```python
from build123d import *

# Parameters (mm, degrees)
F1_DEPTH = 3


with BuildPart() as f1:
    # F0 (on Front) → F1 (new body)
    with BuildSketch(Plane.XZ):
        Polygon((152.04934, 116.75), (152.04934, 119.75), (136.84934, 119.75), (136.84934, 116.75), (121.64934, 116.75), (121.64934, 119.75), (106.44934, 119.75), (106.44934, 116.75), (91.24934, 116.75), (91.24934, 119.75), (76.04934, 119.75), (76.04934, 116.75), (60.84934, 116.75), (60.84934, 119.75), (45.64934, 119.75), (45.64934, 116.75), (30.44934, 116.75), (30.44934, 119.75), (15.24934, 119.75), (15.24934, 116.75), (0.04934, 116.75), (-0.04934, 116.75), (-0.04934, 119.75), (-15.24934, 119.75), (-15.24934, 116.75), (-30.44934, 116.75), (-30.44934, 119.75), (-45.64934, 119.75), (-45.64934, 116.75), (-60.84934, 116.75), (-60.84934, 119.75), (-76.04934, 119.75), (-76.04934, 116.75), (-91.24934, 116.75), (-91.24934, 119.75), (-106.44934, 119.75), (-106.44934, 116.75), (-121.64934, 116.75), (-121.64934, 119.75), (-136.84934, 119.75), (-136.84934, 116.75), (-152.04934, 116.75), (-152.04934, 119.75), (-167.24934, 119.75), (-167.24934, 106.45), (-164.24934, 106.45), (-164.24934, 93.15), (-167.24934, 93.15), (-167.24934, 79.85), (-164.24934, 79.85), (-164.24934, 66.55), (-167.24934, 66.55), (-167.24934, 53.25), (-164.24934, 53.25), (-164.24934, 39.95), (-167.24934, 39.95), (-167.24934, 26.65), (-164.24934, 26.65), (-164.24934, 13.35), (-167.24934, 13.35), (-167.24934, 0.05), (-164.24934, 0.05), (-164.24934, -0.05), (-164.24934, -13.35), (-167.24934, -13.35), (-167.24934, -26.65), (-164.24934, -26.65), (-164.24934, -39.95), (-167.24934, -39.95), (-167.24934, -53.25), (-164.24934, -53.25), (-164.24934, -66.55), (-167.24934, -66.55), (-167.24934, -79.85), (-164.24934, -79.85), (-164.24934, -93.15), (-167.24934, -93.15), (-167.24934, -106.45), (-164.24934, -106.45), (-164.24934, -119.75), (-152.04934, -119.75), (-152.04934, -116.75), (-136.84934, -116.75), (-136.84934, -119.75), (-121.64934, -119.75), (-121.64934, -116.75), (-106.44934, -116.75), (-106.44934, -119.75), (-91.24934, -119.75), (-91.24934, -116.75), (-76.04934, -116.75), (-76.04934, -119.75), (-60.84934, -119.75), (-60.84934, -116.75), (-45.64934, -116.75), (-45.64934, -119.75), (-30.44934, -119.75), (-30.44934, -116.75), (-15.24934, -116.75), (-15.24934, -119.75), (-0.04934, -119.75), (-0.04934, -116.75), (0.04934, -116.75), (15.24934, -116.75), (15.24934, -119.75), (30.44934, -119.75), (30.44934, -116.75), (45.64934, -116.75), (45.64934, -119.75), (60.84934, -119.75), (60.84934, -116.75), (76.04934, -116.75), (76.04934, -119.75), (91.24934, -119.75), (91.24934, -116.75), (106.44934, -116.75), (106.44934, -119.75), (121.64934, -119.75), (121.64934, -116.75), (136.84934, -116.75), (136.84934, -119.75), (152.04934, -119.75), (152.04934, -116.75), (164.24934, -116.75), (164.24934, -106.45), (167.24934, -106.45), (167.24934, -93.15), (164.24934, -93.15), (164.24934, -79.85), (167.24934, -79.85), (167.24934, -66.55), (164.24934, -66.55), (164.24934, -53.25), (167.24934, -53.25), (167.24934, -39.95), (164.24934, -39.95), (164.24934, -26.65), (167.24934, -26.65), (167.24934, -13.35), (164.24934, -13.35), (164.24934, -0.05), (164.24934, 0.05), (167.24934, 0.05), (167.24934, 13.35), (164.24934, 13.35), (164.24934, 26.65), (167.24934, 26.65), (167.24934, 39.95), (164.24934, 39.95), (164.24934, 53.25), (167.24934, 53.25), (167.24934, 66.55), (164.24934, 66.55), (164.24934, 79.85), (167.24934, 79.85), (167.24934, 93.15), (164.24934, 93.15), (164.24934, 106.45), (167.24934, 106.45), (167.24934, 116.75), align=None)
    extrude(amount=F1_DEPTH)


solid = f1.part
```
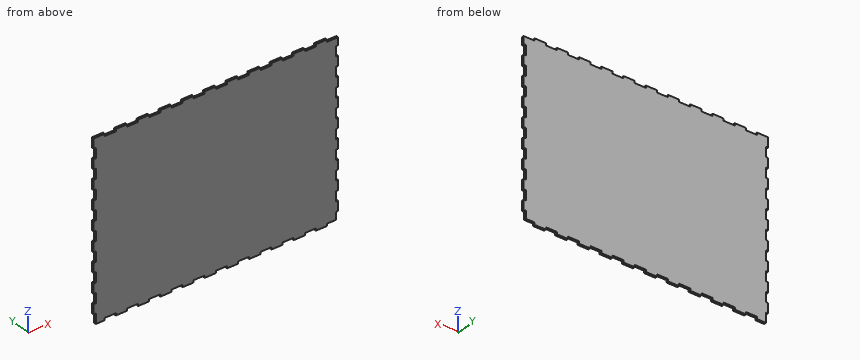
Geometry: final body of the model. Coordinates: model frame, mm. Coordinates: 2 decimals unless noted, no trailing zeros. Loops run counter-clockwise (first coordinate to the right, second up) from the corner with the lowest first, then second, coordinate; pieces in that order, holes last. Notation, with made-up numbers: (48.25, 44) -> (93.25, 44) arc R19 cw to (93.25, 72) -> close; hole circle Ø5 at (-30, 83.5). An arc over 180 degrees is marked (long way). Use a Markdown table: item, result. Add a question column.
(1) Section query A-A, the plane z = -59.5. Return loops of the section in (x, y), plus the area to 3 significant figures.
(2) Pin query (flat end, axial travel): pin 1 Ø1.5 at (x, y) = (-82.5, -1) entering from -Z; pin 2 Ø1.5 at (y, z) = (-2, -119) entering from -X; pin 3 Ø0.9 at (y, z) = (-1, 118) entering from +X. Return the tip coordinate at first contact, or that it passes through.
(3) Line query: line 1 along X through (y, z) = (-1.55, 104.5); line 2 along Z through (x, y) = (-116.5, -2.75). Output: solid intervals per line, ascending.
(4) Section query B-B, the plane x = 66. Return loops of the section in (y, z).
Answer:
| question | item | result |
|---|---|---|
| 1 | outline | (-164.25, -3) -> (164.25, -3) -> (164.25, 0) -> (-164.25, 0) -> close |
| 1 | area | 985 mm^2 |
| 2 | pin 1 | stops at z = -116.75 |
| 2 | pin 2 | stops at x = -164.25 |
| 2 | pin 3 | stops at x = 152.05 |
| 3 | line 1 | x = -164.25 to 164.25 |
| 3 | line 2 | z = -116.75 to 116.75 |
| 4 | outline | (-3, -116.75) -> (0, -116.75) -> (0, 116.75) -> (-3, 116.75) -> close |
